from build123d import *

# Parameters (mm, degrees)
CROQUIS1_R              = 4.445
SALIENTE_EXTRUIR1_DEPTH = 1.905


with BuildPart() as part:
    # Croquis1 → Saliente-Extruir1 (new body)
    with BuildSketch(Plane.XY):
        with BuildLine():
            ThreePointArc((-72.457149103, 51.732991832), (-81.558956176, 37.761513936), (-64.886953379, 37.4625))
            ThreePointArc((-64.886953379, 37.4625), (0, 74.925), (64.886953379, 37.4625))
            ThreePointArc((64.886953379, 37.4625), (81.558956176, 37.761513936), (72.457149103, 51.732991832))
            ThreePointArc((72.457149103, 51.732991832), (44.515, 77.102241699), (8.573510589, 88.616227725))
            ThreePointArc((8.573510589, 88.616227725), (0, 93.985), (-8.573510589, 88.616227725))
            ThreePointArc((-8.573510589, 88.616227725), (-44.515, 77.102241699), (-72.457149103, 51.732991832))
        make_face()
        with Locations((-73.140175477, 42.2275)):
            Circle(CROQUIS1_R, mode=Mode.SUBTRACT)
        with Locations((73.140175477, 42.2275)):
            Circle(CROQUIS1_R, mode=Mode.SUBTRACT)
        with Locations((0, 84.455)):
            Circle(CROQUIS1_R, mode=Mode.SUBTRACT)
    extrude(amount=SALIENTE_EXTRUIR1_DEPTH)


solid = part.part
Read the model definition and answer for the solid it produces. Units are mm, in the model's axes. Give positions to 0.01 mm unless a question says otherwise; leave off trailing zeros. Loops run counter-clockwise (first coordinate to the right, second up) from the corner with the lowest first, then second, coordinate; pieces in that order, holes last. Notation, with made-up numbers: (-7.75, 23.5) - (41.25, 23.5) arc R18 ccw to (41.25, 27.5) - close; hole circle Ø10 at (86, 35.5). An arc over 180 degrees is marked (long way). Answer as CSV lines item,"result". Start each with the question number.
1) Determine the mould class of faces 1 (the face through (-7, 75, 0)), 2 (the face through (0.149, 93.984, 0.939)), 3 (the face through (-77.58, 42.42, 0.94)), 4 (the face through (-81.688, 38.015, 0.939)) for opening direction X: released by +X, released by -X, zero draft, split by the parting line, or undercut.
2) Find section B-B (y = 56). Write down the section's boundary in (x, z) (3 decimals).
3) Find section C-C (z = 1.5). State how many separate pieces and enclosed holes the cut face has, then the cut area to 3 significant figures.
4) Straight lines are drawn through the part: L1, parallel to X at y = 46, z = 1.3; L2, parallel to X at y = 45, z = 0.7; L3, parallel to Y at x = 0, z = 1.65 (3 decimals). For each, find the intervals that lie inside material, in ascending order. Write a range as from..to.
5) Find section D-D (x = -39). Write down the section's boundary in (y, z) (3 decimals).
6) Find section A-A (x = 0). Write down the section's boundary in (y, z) (3 decimals).
Findings below:
1,face 1,"zero draft"
1,face 2,"split by the parting line"
1,face 3,"undercut"
1,face 4,"undercut"
2,outline,"(-69.212, 0) - (-49.777, 0) - (-49.777, 1.905) - (-69.212, 1.905) - close; (49.777, 0) - (69.212, 0) - (69.212, 1.905) - (49.777, 1.905) - close"
3,separate pieces,"1"
3,enclosed holes,"3"
3,area,"2,640 mm^2"
4,L1,"-81.89..-75.49, -70.79..-59.14, 59.14..70.79, 75.49..81.89"
4,L2,"-82.26..-76.61, -69.67..-59.91, 59.91..69.67, 76.61..82.26"
4,L3,"74.925..80.01, 88.9..93.985"
5,outline,"(63.975, 0) - (80.033, 0) - (80.033, 1.905) - (63.975, 1.905) - close"
6,outline,"(74.925, 0) - (80.01, 0) - (80.01, 1.905) - (74.925, 1.905) - close; (88.9, 0) - (93.985, 0) - (93.985, 1.905) - (88.9, 1.905) - close"
